Check sheet for the modelled part. Datum: model origin and axes. Units: mm. Give positions to 0.01 mm unless a question says otherwise; leave off trailing zeros. Order: outer loops, then holes, each group sorted by start corner. A loop starts at its lowest first (then second) coordinate and runs counter-clockwise, first axis right, second up.
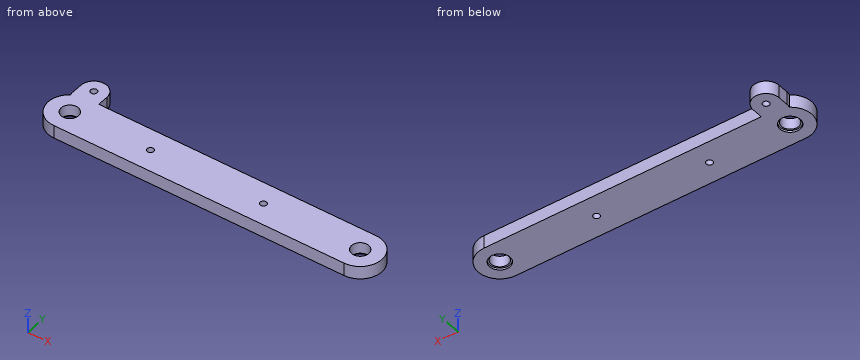
```python
from build123d import *

# Parameters (mm, degrees)
SKETCH_1_R                   = 4
EXTRUDE_1_DEPTH              = 6
HOLE_WIZARD_M5_1_D           = 8
HOLE_WIZARD_M5_1_CBORE_D     = 9.5
HOLE_WIZARD_M5_1_CBORE_DEPTH = 0.9
SKETCH_7_R                   = 1.5
CUT_EXTRUDE_1_DEPTH          = 1
CUT_EXTRUDE_1_DEPTH_BACK     = 7


with BuildPart() as part:
    # 草图1 → 凸台-拉伸1 (new body)
    with BuildSketch(Plane.XY):
        with BuildLine():
            Line((0, 10), (135, 10))
            ThreePointArc((135, 10), (145, 0), (135, -10))
            Line((135, -10), (0, -10))
            ThreePointArc((0, -10), (-10, 0), (0, 10))
        make_face()
        with Locations((135, 0)):
            Circle(SKETCH_1_R, mode=Mode.SUBTRACT)
        Circle(SKETCH_1_R, mode=Mode.SUBTRACT)
        with BuildLine():
            Line((-6, 10), (-6, 15))
            ThreePointArc((-6, 15), (0, 21), (6, 15))
            Line((6, 15), (6, 10))
            ThreePointArc((6, 10), (0, 4), (-6, 10))
        make_face()
    extrude(amount=EXTRUDE_1_DEPTH)

    # M5 六角头螺栓的柱形沉头孔1 (through all)
    with Locations(Plane(origin=(0, 0, 0), x_dir=(-1, 0, 0), z_dir=(0, 0, -1))):
        with Locations((-135, 0), (0, 0)):
            CounterBoreHole(HOLE_WIZARD_M5_1_D / 2, HOLE_WIZARD_M5_1_CBORE_D / 2, HOLE_WIZARD_M5_1_CBORE_DEPTH)

    # 草图7 → 切除-拉伸1 (cut, two sides)
    with BuildSketch(Plane(origin=(0, 0, 0), x_dir=(-1, 0, 0), z_dir=(0, 0, -1))) as cut_extrude_1_sk:
        with Locations((-37.5, 0)):
            Circle(SKETCH_7_R)
        with Locations((-90, 0)):
            Circle(SKETCH_7_R)
        with Locations((0, 15)):
            Circle(SKETCH_7_R)
    extrude(amount=CUT_EXTRUDE_1_DEPTH, mode=Mode.SUBTRACT)
    extrude(cut_extrude_1_sk.sketch, amount=-CUT_EXTRUDE_1_DEPTH_BACK, mode=Mode.SUBTRACT)


solid = part.part
```
(1) Material ranges on L1, parallel to Y at x = 0, z = 0.6; L2, parallel to Y at x = 135, z = 3.95; L3, parallel to Y at x = 135, z = 0.45, recorded low to high.
Response values:
L1: y = -10 to -4.75, 4.75 to 13.5, 16.5 to 21
L2: y = -10 to -4, 4 to 10
L3: y = -10 to -4.75, 4.75 to 10
(2) Cross-section at D-D on x = 109.5. Enter the section's corners in (y, z).
Response values:
outline: (-10, 0) - (10, 0) - (10, 6) - (-10, 6) - close
(3) Cross-section at B-B on x = 90. Enter the section's corners in (y, z), then the cut area to 3 significant figures.
Response values:
outline: (-10, 0) - (-1.5, 0) - (-1.5, 6) - (-10, 6) - close; (1.5, 0) - (10, 0) - (10, 6) - (1.5, 6) - close
area: 102 mm2
(4) Cross-section at A-A on y = 0. Enter the section's corners in (x, z).
Response values:
outline: (-10, 0) - (-4.75, 0) - (-4.75, 0.9) - (-4, 0.9) - (-4, 6) - (-10, 6) - close; (4, 0.9) - (4.75, 0.9) - (4.75, 0) - (36, 0) - (36, 6) - (4, 6) - close; (39, 0) - (88.5, 0) - (88.5, 6) - (39, 6) - close; (91.5, 0) - (130.25, 0) - (130.25, 0.9) - (131, 0.9) - (131, 6) - (91.5, 6) - close; (139, 0.9) - (139.75, 0.9) - (139.75, 0) - (145, 0) - (145, 6) - (139, 6) - close
(5) Gauge pin test, flat ends, axial feed: pin 1 Ø2.5 at (x, y) = (90, 0) entering from -Z; pin 2 Ø3.5 at (x, y) = (0, 15) entering from -Z; pin 3 Ø1.5 at (y, z) = (2.5, 1.5) entering from -X; pin 4 Ø2.5 at (y, z) = (12, 4) entering from -X. Record the tip position at first contact, or that the pin passes through.
Response values:
pin 1: passes through
pin 2: stops at z = 0
pin 3: stops at x = -9.85
pin 4: stops at x = -6
(6) Cross-section at C-C on z = 1.9. Enter the section's corners in (x, y), then the cut area to 3 significant figures.
Response values:
outline: (-6, 10) arc R6 ccw to (-5.72, 8.2) arc R10 ccw to (0, -10) - (135, -10) arc R10 ccw to (135, 10) - (6, 10) - (6, 15) arc R6 ccw to (-6, 15) - close; hole circle Ø8 at (0, 0); hole circle Ø3 at (0, 15); hole circle Ø3 at (37.5, 0); hole circle Ø3 at (90, 0); hole circle Ø8 at (135, 0)
area: 3,010 mm2
